Read the model definition and answer for the solid it produces. Units are mm, in the model's axes. Round coordinates to 2 decimals unless told otherwise and drop trailing zeros. Loops run counter-clockwise (first coordinate to the right, second up) from the corner with the lowest first, then second, coordinate; pieces in that order, holes last. Notation, with made-up numbers: (55, 73) -> (69, 73) arc R22 cw to (69, 105) -> close; hole circle Ø3 at (68, 35). An arc over 180 degrees is marked (long way). Put each result on its own line as item: value.
Autodesk Inventor part; units mm, degrees
ref_plane "YZ Plane" through (0, 0, 0) normal (1, 0, 0) x (0, 1, 0)
ref_plane "XZ Plane" through (0, 0, 0) normal (0, 1, 0) x (-1, 0, 0)
ref_plane "XY Plane" through (0, 0, 0) normal (0, 0, 1) x (1, 0, 0)
sketch "Эскиз1" plane through (0, 0, 0) normal (0, 0, 1) x (1, 0, 0)
  circle A0 centre (0, 0) radius 4
  line L0 (8.0829, 0) -> (4.0415, -7)
  line L1 (4.0415, -7) -> (-4.0415, -7)
  line L2 (-4.0415, -7) -> (-8.0829, 0)
  line L3 (-8.0829, 0) -> (-4.0415, 7)
  line L4 (-4.0415, 7) -> (4.0415, 7)
  line L5 (4.0415, 7) -> (8.0829, 0)
  dimension "d0" = 8
  dimension "d1" = 14
extrude "Выдавливание1" add sketch "Эскиз1" along normal blind 4
sketch "Эскиз2" plane through (0, 0, 0) normal (0, 1, 0) x (-1, 0, 0)
  line L0 (0, 0) -> (0, 12.9838)
  line L1 (-4.0415, 0) -> (-8.0829, 0) construction
  line L2 (-8.0829, 0) -> (-8.0829, 4) construction
  line L3 (-8.0829, 4) -> (-4.0415, 4) construction
  line L4 (-3.7273, -1.9581) -> (-10.5829, 2)
  line L5 (-10.5829, 2) -> (-3.7273, 5.9581)
  line L6 (-3.7273, 5.9581) -> (-11.5829, 5.9581)
  line L7 (-11.5829, 5.9581) -> (-11.5829, -1.9581)
  line L8 (-11.5829, -1.9581) -> (-3.7273, -1.9581)
  line L9 (-8.0829, 2) -> (-29.2681, 2) construction
  point P0 (-11.5829, 2)
  dimension "d4" = 60
  dimension "d5" = 1
  dimension "d6" = 3.5
revolve "Вращение1" cut sketch "Эскиз2" angle 360 about axis through (0, 0, 0) along (0, 0, 1)
sketch "Эскиз3" plane through (0, 0, 0) normal (0, 0, -1) x (-1, 0, 0)
  line L0 (5.4146, -4.6216) -> (6.7097, -2.3784) construction
  circle A0 centre (0, 0) radius 7
  circle A1 centre (0, 0) radius 4
extrude "Выдавливание2" add sketch "Эскиз3" along normal blind 3
fillet "Сопряжение1" radius 2 1 edges at (7, 0, -3)
sketch "Эскиз4" plane through (0, 0, -3) normal (0, 0, -1) x (-1, 0, 0)
  circle A0 centre (0, 0) radius 4
  circle A1 centre (0, 0) radius 4.65
  dimension "d14" = 9.3
extrude "Выдавливание3" cut sketch "Эскиз4" against normal blind 0.2
fillet "Сопряжение2" radius 0.2 1 edges at (4.65, 0, -3)
chamfer "Фаска2" distance 0.5 angle 45 1 edges at (-4, 0, 4)
properties part number "paris_nut"
Item 1: The part is cut by section A-A (z = 1.75). Determine the outline of the cut face in (x, y).
Derived:
outline: (-8.08, 0) -> (-4.04, -7) -> (4.04, -7) -> (8.08, 0) -> (4.04, 7) -> (-4.04, 7) -> close; hole circle Ø8 at (0, 0)
Item 2: The part is cut by section B-B (z = -1.75). Determine the outline of the cut face in (x, y).
Derived:
outline: circle Ø13.71 at (0, 0); hole circle Ø8 at (0, 0)
Item 3: For a pull along X with two mould halves and no side action, classify faces 1 (the cylindrical face through (-6.466, 2.681, -0.493)), 2 (the conical face through (-3.73, -6.39, 0.16)), 3 (the flat face through (0, -7, 2)), 4 (the conical face through (3.73, 6.39, 0.16)) as pulls with the +X half, pulls with the -X half, needs draft (parallel to the pull), parting line crosses it, or undercut.
Derived:
face 1: parting line crosses it
face 2: pulls with the -X half
face 3: needs draft
face 4: pulls with the +X half
Item 4: Flat-ended cylindrical pins translate along their axes: pin 1 Ø2 at (x, y) = (-3, 5.5) entering from -Z; pin 2 Ø1.5 at (y, z) = (-3.5, 2.5) entering from +X. Find the tip coordinate at first contact, or state that the pin passes through.
Derived:
pin 1: stops at z = -2.98
pin 2: stops at x = 6.5
Item 5: Find the intervals of material crossed by line 1 along Y through (x, z) = (0, 2.2); line 2 along Y through (x, z) = (-5.75, 1.25), in increasing order.
Derived:
line 1: y = -7 to -4, 4 to 7
line 2: y = -4.04 to 4.04
